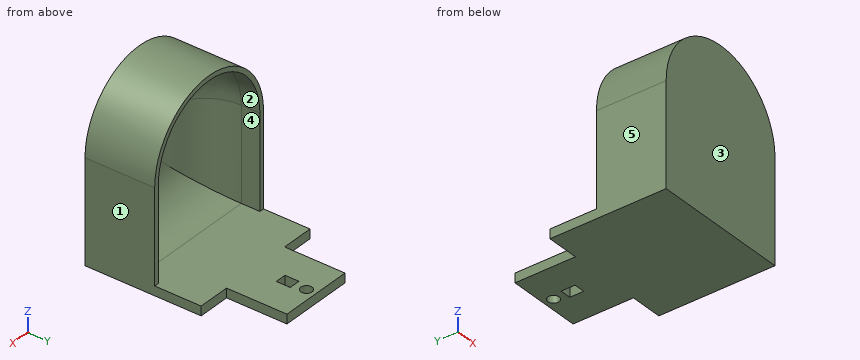
from build123d import *

# Parameters (mm, degrees)
BOSS_EXTRUDE1_DEPTH = 1.27
BOSS_EXTRUDE3_DEPTH = 17.78
SKETCH5_W           = 38.1
SKETCH5_H           = 19.05
BOSS_EXTRUDE4_DEPTH = 2.54
FILLET1_R           = 12.7
BOSS_EXTRUDE5_DEPTH = 2.54
CUT_EXTRUDE6_REACH  = 48.99
SKETCH12_R          = 1.524
SKETCH12_W          = 3.048
SKETCH12_H          = 3.81


with BuildPart() as part:
    # Sketch1 → Boss-Extrude1 (new body)
    with BuildSketch(Plane(origin=(0, 0, 0), x_dir=(1, 0, 0), z_dir=(0, 1, 0))):
        with BuildLine():
            Line((0, 0), (38.1, 0))
            Line((38.1, 0), (38.1, -25.4))
            ThreePointArc((38.1, -25.4), (19.05, -44.45), (0, -25.4))
            Line((0, -25.4), (0, 0))
        make_face()
    extrude(amount=BOSS_EXTRUDE1_DEPTH)

    # Sketch3 → Boss-Extrude3 (add)
    with BuildSketch(Plane(origin=(0, 1.27, 0), x_dir=(1, 0, 0), z_dir=(0, 1, 0))):
        with BuildLine():
            Line((0, 0), (0, -25.4))
            ThreePointArc((0, -25.4), (19.05, -44.45), (38.1, -25.4))
            Line((38.1, -25.4), (38.1, 0))
            Line((38.1, 0), (36.83, 0))
            Line((36.83, 0), (36.83, -25.4))
            ThreePointArc((36.83, -25.4), (19.05, -43.18), (1.27, -25.4))
            Line((1.27, -25.4), (1.27, 0))
            Line((1.27, 0), (0, 0))
        make_face()
    extrude(amount=BOSS_EXTRUDE3_DEPTH)

    # Sketch5 → Boss-Extrude4 (add)
    with BuildSketch(Plane(origin=(0, 0, 0), x_dir=(-1, 0, 0), z_dir=(0, 0, -1))):
        with Locations((-19.05, 9.525)):
            Rectangle(SKETCH5_W, SKETCH5_H)
    extrude(amount=BOSS_EXTRUDE4_DEPTH)

    # Fillet1
    fillet1_edges = [part.edges().sort_by_distance(p)[0] for p in [
        (19.05, 1.27, 0),
        (36.83, 1.27, 12.7),
        (19.05, 1.27, 43.18),
        (1.27, 1.27, 12.7),
    ]]
    fillet(fillet1_edges, radius=FILLET1_R)

    # Sketch10 → Boss-Extrude5 (add)
    with BuildSketch(Plane(origin=(0, 0, -2.54), x_dir=(-1, 0, 0), z_dir=(0, 0, -1))):
        Polygon((-29.21, 31.75), (-29.21, 48.26), (-8.89, 48.26), (-8.89, 31.75), (0, 31.75), (0, 19.05), (-38.1, 19.05), (-38.1, 31.75), align=None)
    extrude(amount=-BOSS_EXTRUDE5_DEPTH)

    # Sketch12 → Cut-Extrude6 (cut, up to next)
    with BuildSketch(Plane(origin=(0, 0, -2.54), x_dir=(-1, 0, 0), z_dir=(0, 0, -1)), mode=Mode.PRIVATE) as cut_extrude6_sk1:
        with Locations((-19.05, 45.6565)):
            Circle(SKETCH12_R)
    cut_extrude6_tool1 = extrude(cut_extrude6_sk1.sketch, amount=-CUT_EXTRUDE6_REACH, mode=Mode.PRIVATE) & part.part
    add(cut_extrude6_tool1.solids().sort_by_distance((19.05, 45.6565, -2.54))[0], mode=Mode.SUBTRACT)
    # Sketch12 → Cut-Extrude6 (cut, up to next)
    with BuildSketch(Plane(origin=(0, 0, -2.54), x_dir=(-1, 0, 0), z_dir=(0, 0, -1)), mode=Mode.PRIVATE) as cut_extrude6_sk2:
        with Locations((-19.05, 40.513)):
            Rectangle(SKETCH12_W, SKETCH12_H)
    cut_extrude6_tool2 = extrude(cut_extrude6_sk2.sketch, amount=-CUT_EXTRUDE6_REACH, mode=Mode.PRIVATE) & part.part
    add(cut_extrude6_tool2.solids().sort_by_distance((19.05, 40.513, -2.54))[0], mode=Mode.SUBTRACT)


solid = part.part
Here's how the part is built. I have some questions about the finished solid (model axes, mm). Face numbers are marked on the shaded views. A direction names the side the tool comes from. Coordinates: 2 decimals unless noted, no trailing zeros. Write each loop counter-clockwise with the first axis right and the second up, starting at its lowest first coordinate (ties: lowest second). Pieces come first, ordered by that corner, then holes.
Item 1: If we mould it in two halves opening along X, with no side actions, what happens to the marked faces 3, 4 and 5? For each: +X half, -X half, draft (parallel to the pull), parting line (faces both ways), or undercut.
Item 2: On a 3-axis mill with a long thin cutter (end or side, diameter ignored), from which of +Z, -Z, +X, -X, +Y, -Y can I reach the whole of each face in a straight line? I mean the marked faces 1 and 2. Say none if no direction works.
Item 3: I want a section at B-B on y = 16. Write out the boundary of the cut face in (x, z).
Item 4: I want a section at D-D on z = 3. Write out the boundary of the cut face in (x, y), and give its area (3 significant figures).
Item 5: I want a section at C-C on x = 19.05. Count the separate pieces of the cut face and the enclosed holes in it, and give its area (3 significant figures).
Item 6: I want a section at A-A on y = 39.5. Write out the boundary of the cut face in (x, z), and give its area (3 significant figures).
Item 7: Will these pins go through, and if not, where does the flat tip stop? pin 1 (0.8 mm diameter, centred on y = 39, z = -1.5, fed in from -X); pin 2 (4 mm diameter, centred on x = 9, z = 23.5, fed in from +Y); pin 3 (11.5 mm diameter, centred on x = 12.5, z = 16, fed in from +Y).
Item 8: If I drill on line 1 (Y direction, x = 19.05, z = -1.4); line 2 (X direction, y = 19, z = 1); line 3 (Z direction, x = 15, y = 20.5), over which ranges is the centre line in solid material (lowest first)?
Findings below:
1. face 3: draft
1. face 4: undercut
1. face 5: -X half
2. face 1: +Z, -Z, +X, +Y, -Y
2. face 2: +Y
3. outline: (0, -2.54) - (38.1, -2.54) - (38.1, 25.4) arc R19.05 ccw to (0, 25.4) - close; hole (1.27, 0) - (36.83, 0) - (36.83, 25.4) arc R17.78 ccw to (1.27, 25.4) - close
4. outline: (0, 0) - (38.1, 0) - (38.1, 19.05) - (36.83, 19.05) - (36.83, 13.97) arc R12.7 cw to (33.83, 5.77) - (4.27, 5.77) arc R12.7 cw to (1.27, 13.97) - (1.27, 19.05) - (0, 19.05) - close
4. area: 269 mm2
5. separate pieces: 3
5. enclosed holes: 0
5. area: 253 mm2
6. outline: (8.89, -2.54) - (17.53, -2.54) - (17.53, 0) - (8.89, 0) - close; (20.57, -2.54) - (29.21, -2.54) - (29.21, 0) - (20.57, 0) - close
6. area: 43.9 mm2
7. pin 1: stops at x = 8.89
7. pin 2: stops at y = 3.35
7. pin 3: stops at y = 3.52
8. line 1: y = 0 to 38.61, 42.42 to 44.13, 47.18 to 48.26
8. line 2: x = 0 to 1.27, 36.83 to 38.1
8. line 3: z = -2.54 to 0
